from build123d import *

# Parameters (mm, degrees)
F0_R     = 40.64
F1_DEPTH = 3.81
F3_DEPTH = 25.4
F4_R     = 8.89
F5_DEPTH = 7.62
F7_DEPTH = 6.35
F8_R     = 2.159
F9_DEPTH = 25.4


with BuildPart() as f1:
    # F0 (on Front) → F1 (new body)
    with BuildSketch(Plane.XZ):
        Circle(F0_R)
    extrude(amount=F1_DEPTH)

    # F2 (on face) → F3 (cut)
    with BuildSketch(Plane.XZ.offset(3.81)):
        with BuildLine():
            Line((-30.206892, 7.62), (-7.62, 7.62))
            Line((-7.62, 7.62), (-7.62, 30.206892))
            ThreePointArc((-7.62, 30.206892), (-10.132805, 34.590488), (-15.185319, 34.637421))
            ThreePointArc((-15.185319, 34.637421), (-26.253153, 26.253153), (-34.637421, 15.185319))
            ThreePointArc((-34.637421, 15.185319), (-34.590488, 10.132805), (-30.206892, 7.62))
        make_face()
        with BuildLine():
            Line((-16.581494, -26.373752), (-9.60176, -4.892341))
            Line((-9.60176, -4.892341), (-31.083171, 2.087392))
            ThreePointArc((-31.083171, 2.087392), (-36.028718, 1.052178), (-37.634667, -3.738545))
            ThreePointArc((-37.634667, -3.738545), (-33.080903, -16.855562), (-25.145648, -28.249624))
            ThreePointArc((-25.145648, -28.249624), (-20.325919, -29.7663), (-16.581494, -26.373752))
        make_face()
        with BuildLine():
            ThreePointArc((-11.590456, -28.916813), (-12.134167, -33.940206), (-8.074184, -36.947969))
            ThreePointArc((-8.074184, -36.947969), (5.808031, -36.670464), (19.096556, -32.644547))
            ThreePointArc((19.096556, -32.644547), (22.028379, -28.52939), (19.958965, -23.919875))
            Line((19.958965, -23.919875), (1.685786, -10.643633))
            Line((1.685786, -10.643633), (-11.590456, -28.916813))
        make_face()
        with BuildLine():
            ThreePointArc((23.919875, -19.958965), (28.52939, -22.028379), (32.644547, -19.096556))
            ThreePointArc((32.644547, -19.096556), (36.670464, -5.808031), (36.947969, 8.074184))
            ThreePointArc((36.947969, 8.074184), (33.940206, 12.134167), (28.916813, 11.590456))
            Line((28.916813, 11.590456), (10.643633, -1.685786))
            Line((10.643633, -1.685786), (23.919875, -19.958965))
        make_face()
        with BuildLine():
            ThreePointArc((26.373752, 16.581494), (29.7663, 20.325919), (28.249624, 25.145648))
            ThreePointArc((28.249624, 25.145648), (16.855562, 33.080903), (3.738545, 37.634667))
            ThreePointArc((3.738545, 37.634667), (-1.052178, 36.028718), (-2.087392, 31.083171))
            Line((-2.087392, 31.083171), (4.892341, 9.60176))
            Line((4.892341, 9.60176), (26.373752, 16.581494))
        make_face()
    extrude(amount=-F3_DEPTH, mode=Mode.SUBTRACT)

    # F4 (on face) → F5 (join)
    with BuildSketch(Plane.XZ.offset(3.81)):
        Circle(F4_R)
    extrude(amount=F5_DEPTH)

    # F6 (on face) → F7 (cut)
    with BuildSketch(Plane.XZ.offset(11.43)):
        Polygon((3.519527, -6.096), (7.039054, 0), (3.519527, 6.096), (-3.519527, 6.096), (-7.039054, 0), (-3.519527, -6.096), align=None)
    extrude(amount=-F7_DEPTH, mode=Mode.SUBTRACT)

    # F8 (on face) → F9 (cut)
    with BuildSketch(Plane.XZ.offset(5.08)):
        Circle(F8_R)
    extrude(amount=-F9_DEPTH, mode=Mode.SUBTRACT)

    # F10 (on Top) → F11 (revolve, cut)
    with BuildSketch(Plane.XY):
        with BuildLine():
            Line((40.64, -3.302), (40.64, -0.791535))
            ThreePointArc((40.64, -0.791535), (39.563109, -2.046767), (40.64, -3.302))
        make_face()
    revolve(axis=Axis((0, -1.905, 0), (0, -1, 0)), mode=Mode.SUBTRACT)


solid = f1.part
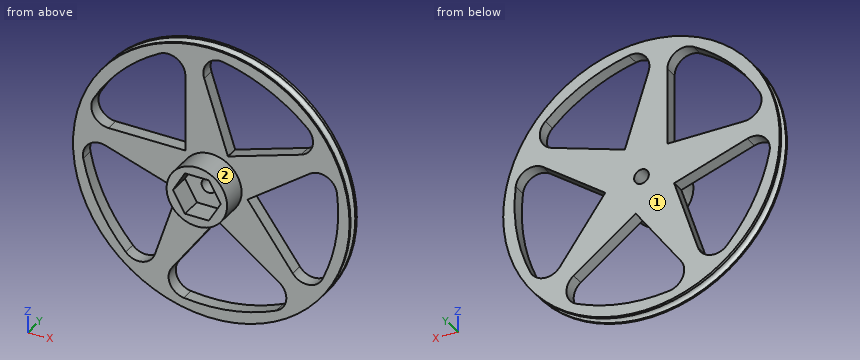
Read the model definition and answer for the solid it produces. Units are mm, in the model's axes. Face numbers are marked on the shaded views. A direction names the side the tool comes from. Coordinates: 2 decimals unless noted, no trailing zeros. Loops run counter-clockwise (first coordinate to the right, second up) from the corner with the lowest first, then second, coordinate; pieces in that order, holes last.
Q1. Which of the six approach directions +Z, -Z, +X, -X, +Y, -Y give full straight-line access (tool end or side, diameter ignored) to the marked faces 1 and 2?
Q2. Each of these flat-tipped pins is pushed along its axis until it touches: pin 1 Ø1.9 at (x, y) = (-1.5, -8) entering from -Z; pin 2 Ø4 at (y, z) = (-3, 15) entering from -X; pin 3 Ø7 at (x, z) = (0, 0) entering from -Y; pin 4 Ø1.5 at (x, z) = (-29, 31.5) entering from +Y. Where does it stop, or does it pass through?
Q3. Consider probe 1 along Z at (x, y) = (0, -4); probe 2 along Z at (x, y) = (0, -11); probe 3 along Y at (x, z) = (19, 34). Determine where each line is inside the solid, lowest interval first.
Q4. The part is cut by section A-A on y = -9. Write down the section's boundary in (x, z), and give its area (3 significant figures).
Q5. The part is cut by section B-B on x = 0. Write down the section's boundary in (y, z), and give its area (3 significant figures).
Q6. The part is cut by section C-C on z = 27. Give the number of separate pieces and of enclosed holes in the cut face, and give its area (3 significant figures).
Results below:
1. face 1: +Z, -Z, +X, -X, +Y
1. face 2: -Y
2. pin 1: stops at z = -8.87
2. pin 2: stops at x = -38.5
2. pin 3: stops at y = -5.08
2. pin 4: passes through
3. probe 1: z = -8.89 to -2.16, 2.16 to 8.89
3. probe 2: z = -8.89 to -6.1, 6.1 to 8.89
3. probe 3: y = -3.81 to 0
4. outline: circle Ø17.78 at (0, 0); hole (-7.04, 0) - (-3.52, -6.1) - (3.52, -6.1) - (7.04, 0) - (3.52, 6.1) - (-3.52, 6.1) - close
4. area: 120 mm2
5. outline: (-11.43, -8.89) - (-3.81, -8.89) - (-3.81, -12.96) - (0, -12.96) - (0, -2.16) - (-5.08, -2.16) - (-5.08, -6.1) - (-11.43, -6.1) - close; (-11.43, 6.1) - (-5.08, 6.1) - (-5.08, 2.16) - (0, 2.16) - (0, 24.66) - (-3.81, 24.66) - (-3.81, 8.89) - (-11.43, 8.89) - close; (-3.81, -40.64) - (-3.3, -40.64) arc R1.27 cw to (-0.79, -40.64) - (0, -40.64) - (0, -37.25) - (-3.81, -37.25) - close; (-3.81, 36.93) - (0, 36.93) - (0, 40.64) - (-0.79, 40.64) arc R1.27 cw to (-3.3, 40.64) - (-3.81, 40.64) - close
5. area: 202 mm2
6. separate pieces: 3
6. enclosed holes: 0
6. area: 55.4 mm2
